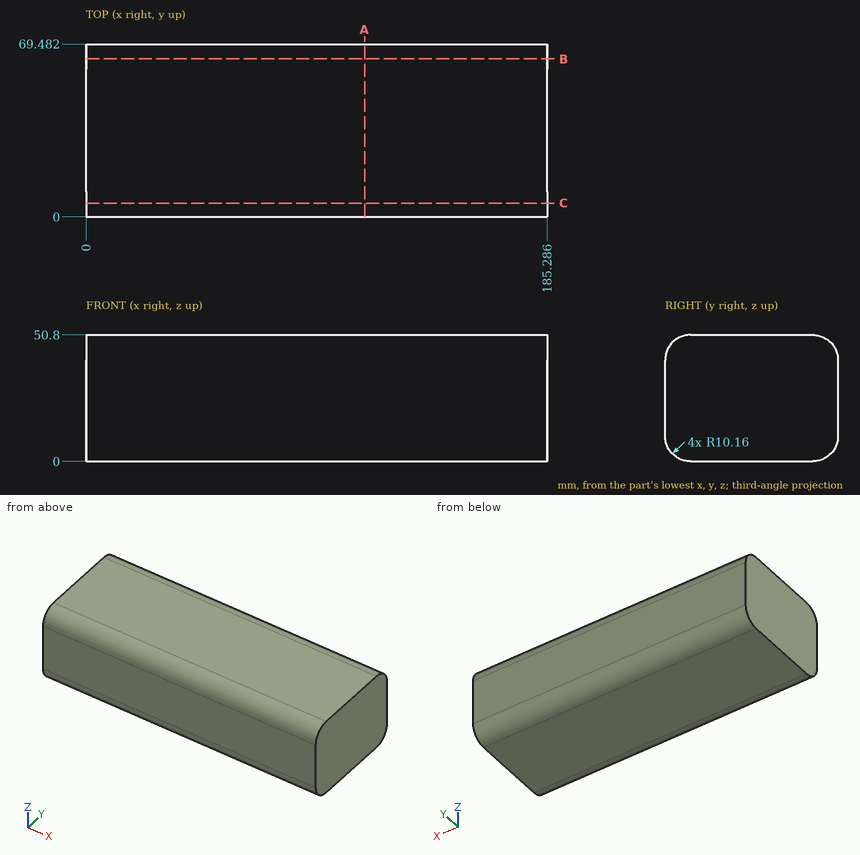
Input: dimensioned drawing with shaded views. Units: mm. Origin: part minimum x, y, z. Round coordinates to 2 decimals unless told otherwise and drop trailing zeros. Loops run counter-clockwise (first coordinate to the right, second up) from the corner with the lowest first, then second, coordinate; pieces in that order, holes last. Notation, with made-up numbers: M 44.25,23 L 75.25,23 A26 cw 75.25,40 Z; hole C 8,5 d11. An arc over 180 degrees is marked long. Answer in a Markdown table with one row per item. Add a question column.
1. Section C-C (y = 5.5). Output: boundary loops of the cut face in (x, z).
2. Contact query for a flat-ended pin moving along its axis: pin 1 (4 mm diameter, centred on x = 127, y = 47, fed in from -Z). Output: stop coordinate, or through.
3. Section A-A (x = 112). Output: boundary loops of the cut face in (y, z), and give its area (3 significant figures).
4. Ray query, probe 1 along Z at (x, y) = (113, 10); probe 2 along Y at (x, z) = (103.5, 43.5); probe 3 along Y at (x, z) = (108, 44). Return the intervals inside material, ascending.
5. Section B-B (y = 63.5). Output: boundary loops of the cut face in (x, z), and give its area (3 significant figures).
Values follow:
| question | item | result |
|---|---|---|
| 1 | outline | M 0,1.13 L 185.29,1.13 L 185.29,49.67 L 0,49.67 Z |
| 2 | pin 1 | z = 0 |
| 3 | outline | M 0,10.16 A10.16 ccw 10.16,0 L 59.32,0 A10.16 ccw 69.48,10.16 L 69.48,40.64 A10.16 ccw 59.32,50.8 L 10.16,50.8 A10.16 ccw 0,40.64 Z |
| 3 | area | 3,440 mm^2 |
| 4 | probe 1 | 0 to 50.8 |
| 4 | probe 2 | 0.41 to 69.07 |
| 4 | probe 3 | 0.57 to 68.91 |
| 5 | outline | M 0,0.9 L 185.29,0.9 L 185.29,49.9 L 0,49.9 Z |
| 5 | area | 9,080 mm^2 |
